```python
from build123d import *

# Parameters (mm, degrees)
BOSS_EXTRUDE1_DEPTH = 5
FILLET1_R           = 5
SKETCH2_R           = 1.3
CUT_EXTRUDE1_DEPTH  = 10
BOSS_EXTRUDE2_DEPTH = 45
BOSS_EXTRUDE3_DEPTH = 15
BOSS_EXTRUDE4_DEPTH = 6
BOSS_EXTRUDE5_START = -5.9
SKETCH6_R           = 4.9
SKETCH6_R_2         = 1.3
BOSS_EXTRUDE5_DEPTH = 5.9
BOSS_EXTRUDE6_DEPTH = 4
BOSS_EXTRUDE7_DEPTH = 5
BOSS_EXTRUDE8_DEPTH = 9
CHAMFER1_SIZE       = 5
FILLET2_R           = 6
SKETCH11_R          = 1.6
CUT_EXTRUDE2_DEPTH  = 10
FILLET3_R           = 10


# Some blends are built 0.0001 mm under size
with BuildPart() as part:
    # Sketch1 → Boss-Extrude1 (new body)
    with BuildSketch(Plane(origin=(0, 0, 0), x_dir=(1, 0, 0), z_dir=(0, 1, 0))):
        Polygon((4.09199016, 5.61187779), (0, 10), (0, 1.796035233), align=None)
        Polygon((0, 1.796035233), (0, 10), (-42.418514694, -29.555904884), (-38.326524534, -33.944027093), (-1.926011986, 0), align=None)
        Polygon((42, 10), (0, 10), (4.09199016, 5.61187779), (0, 1.796035233), (0, 0), (42, 0), align=None)
        Polygon((0, 0), (0, 1.796035233), (-1.926011986, 0), align=None)
    extrude(amount=BOSS_EXTRUDE1_DEPTH)

    # Fillet1
    fillet1_edges = [part.edges().sort_by_distance(p)[0] for p in [
        (42, 2.5, 0),
        (42, 2.5, -10),
    ]]
    fillet(fillet1_edges, radius=FILLET1_R - 0.0001)  # a hair under: the kernel refuses the full size

    # Sketch2 → Cut-Extrude1 (cut)
    with BuildSketch(Plane(origin=(0, 5, 0), x_dir=(1, 0, 0), z_dir=(0, 1, 0))):
        with Locations(Location((37, 5, 0), (0, 0, 270))):
            Circle(SKETCH2_R)
    extrude(amount=-CUT_EXTRUDE1_DEPTH, mode=Mode.SUBTRACT)

    # Sketch3 → Boss-Extrude2 (add)
    with BuildSketch(Plane(origin=(0, 5, 0), x_dir=(1, 0, 0), z_dir=(0, 1, 0))):
        Polygon((-42.418514694, -29.555904884), (-38.326524534, -33.944027093), (-20.12626826, -16.972013547), (-24.21825842, -12.583891337), align=None)
    extrude(amount=BOSS_EXTRUDE2_DEPTH)

    # Sketch4 → Boss-Extrude3 (add)
    with BuildSketch(Plane.XZ):
        Polygon((-42.418514694, 29.555904884), (-38.326524534, 33.944027093), (-20.12626826, 16.972013547), (-24.21825842, 12.583891337), align=None)
    extrude(amount=BOSS_EXTRUDE3_DEPTH)

    # Sketch5 → Boss-Extrude4 (add)
    with BuildSketch(Plane(origin=(-4.987820251, 0, -5.348782369), x_dir=(-0.7313537016191739, 0, 0.6819983600624947), z_dir=(-0.6819983600624948, 0, -0.731353701619174))):
        Polygon((26.294306197, -15), (26.294306197, 0), (13.888976828, 0), align=None)
        Polygon((13.888976828, 5), (26.294306197, 50), (26.294306197, 5), align=None)
    extrude(amount=-BOSS_EXTRUDE4_DEPTH)

    # Sketch6 → Boss-Extrude5 (add)
    with BuildSketch(Plane.XZ.offset(BOSS_EXTRUDE5_START)):
        with Locations(Location((37, -5, 0), (0, 0, 270))):
            Circle(SKETCH6_R)
        with Locations(Location((37, -5, 0), (0, 0, 90))):
            Circle(SKETCH6_R_2, mode=Mode.SUBTRACT)
    extrude(amount=BOSS_EXTRUDE5_DEPTH)

    # Sketch8 → Boss-Extrude6 (add)
    with BuildSketch(Plane.XZ):
        Polygon((0, -10), (-19.681916643, 8.353684194), (-15.589926483, 12.741806404), (8.797675114, -10), align=None)
    extrude(amount=BOSS_EXTRUDE6_DEPTH)

    # Sketch10 → Boss-Extrude7 (add)
    with BuildSketch(Plane(origin=(0, 5, 0), x_dir=(1, 0, 0), z_dir=(0, 1, 0))):
        Polygon((8.797675114, 10), (8.797675114, 0), (-1.926011986, 0), (-16.799617624, -13.869861642), (-20.891607784, -9.481739432), (0, 10), align=None)
    extrude(amount=BOSS_EXTRUDE7_DEPTH)

    # Sketch9 → Boss-Extrude8 (add)
    with BuildSketch(Plane(origin=(0, 5, 0), x_dir=(1, 0, 0), z_dir=(0, 1, 0))):
        Polygon((17.950520425, 10), (8.797675114, 10), (-1.926011986, 0), (8.797675114, 0), (17.950520425, 0), align=None)
    extrude(amount=-BOSS_EXTRUDE8_DEPTH)

    # Chamfer1
    # the kernel refuses this chamfer: 5 mm, written as the material it adds along each edge
    # the kernel refuses this chamfer: 5 mm, written as the material it takes off along each edge
    with BuildSketch(Plane(origin=(17.950520425, -4, 12.85841494), x_dir=(0.027495876610586317, 0.9996219169112968, 0), z_dir=(0, 0, -1))) as chamfer1_2_piece_1_section:
        Polygon((CHAMFER1_SIZE * 0.999621916911, -CHAMFER1_SIZE * 0.0274958766106), (-CHAMFER1_SIZE * 0.0274958766106, -CHAMFER1_SIZE * 0.999621916911), (0, 0), align=None)
    chamfer1_2_piece_1 = extrude(amount=35.71682988, mode=Mode.PRIVATE)
    chamfer1_2_piece_1 = split(chamfer1_2_piece_1, bisect_by=Plane(origin=(16.228298203, 0, -5), z_dir=(0, -1, 0)), keep=Keep.TOP, mode=Mode.PRIVATE)
    add(chamfer1_2_piece_1, mode=Mode.SUBTRACT)

    # Fillet2
    fillet2_edges = [part.edges().sort_by_distance(p)[0] for p in [
        (12.950520425, -4, -5),
        (16.950520425, 0, -5),
    ]]
    fillet(fillet2_edges, radius=FILLET2_R)

    # Sketch11 → Cut-Extrude2 (cut)
    with BuildSketch(Plane(origin=(0, 5, 0), x_dir=(1, 0, 0), z_dir=(0, 1, 0))):
        with Locations(Location((13.5, 5, 0), (0, 0, 270))):
            Circle(SKETCH11_R)
    extrude(amount=-CUT_EXTRUDE2_DEPTH, mode=Mode.SUBTRACT)

    # Fillet3
    fillet3_edges = [part.edges().sort_by_distance(p)[0] for p in [
        (-14.107655737, 10, 7.257584188),
        (-1.926011986, 3, 0),
        (0, 3, -10),
        (-15.518962067, -4, 8.573648632),
    ]]
    fillet(fillet3_edges, radius=FILLET3_R)


solid = part.part
```
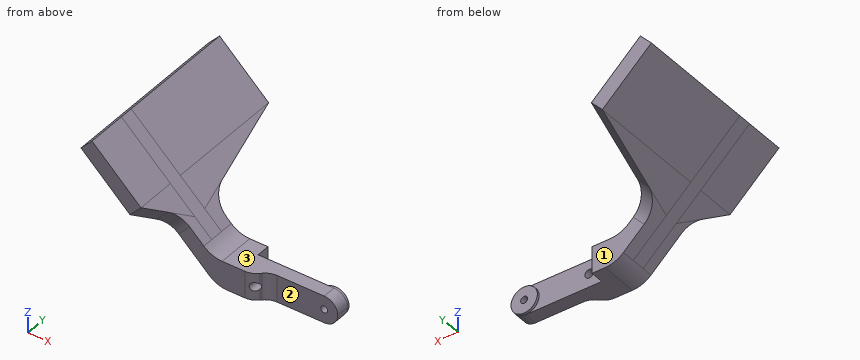
The model under review builds one solid part; all positions refer to its coordinate system, in mm. Face numbers are marked on the shaded views. A direction names the side the tool comes from. Give positions to 0.01 mm unless a question says otherwise; leave off trailing zeros. Loops run counter-clockwise (first coordinate to the right, second up) from the corner with the lowest first, then second, coordinate; pieces in that order, holes last. Notation, with made-up numbers: (36, 68) -> (40, 68) arc R21 ccw to (40, 101) -> close; hole circle Ø1 at (9, 14). An arc over 180 degrees is marked (long way). Use CSV: the item, a comma, the result in double quotes.
1. Consider section B-B, the plane z = 14.5. Write out the cut boundary in (x, y), then the cut area to 3 significant figures.
Result:
outline,"(-26.27, -15) -> (-22.43, -15) -> (-17.48, -10.62) -> (-17.48, 36.85) -> (-22.43, 50) -> (-26.27, 50) -> close"
area,"528 mm²"
2. Machinability: for the marked faces 1, 2 and 3, which of the approach directions +Z, -Z, +X, -X, +Y, -Y give a long, thin tool a straight path to every point of the face, cutting with its end or side? Answer none if there is none.
Result:
face 1,"-Z, +X, +Y"
face 2,"+Z, -Z, +X, -Y"
face 3,"+Z, +X, +Y, -Y"
3. Consider section A-A, the plane x = 13.5. Write out the cut boundary in (y, z), then the cut area to 3 significant figures.
Result:
outline,"(-3.18, -10) -> (5, -10) -> (5, -6.6) -> (-3.18, -6.6) -> close; (-3.18, -3.4) -> (5, -3.4) -> (5, 0) -> (-3.18, 0) -> close"
area,"55.6 mm²"
4. For P1, Ø9, axis at x = 1, z = -1.5, coming from the -Y side; P2, Ø3, axis at x = 30.5, z = -6, coming from the -Y side; P3, Ø2.5, axis at x = 37, z = -5, coming from the +Y side; P4, Ø8, axis at x = 23.5, z = -6, coming from the +Y side, all flat-tipped, find the tip position at first contact; note any pin that passes through.
Result:
P1,"stops at y = -4"
P2,"stops at y = 0"
P3,"passes through"
P4,"stops at y = 5"
5. Consider section C-C, the plane y = 15.5. Write out the cut boundary in (x, z), then the cut area to 3 significant figures.
Result:
outline,"(-42.42, 29.56) -> (-17.11, 5.96) -> (-13.02, 10.35) -> (-38.33, 33.94) -> close"
area,"208 mm²"
6. Consider section D-D, the plane x = 29. Write out the cut boundary in (y, z), then the cut area to 3 significant figures.
Result:
outline,"(0, -10) -> (5, -10) -> (5, 0) -> (0, 0) -> close"
area,"50.0 mm²"
7. To check wall thickness, follow probe 1 along Z at (x, y) = (37, 3.8); probe 2 along X at (y, z) = (3.2, -5); probe 3 along Z at (x, y) = (13.5, 0.5). State the ranges of each line that lie inside material, in increasing order. Write a range as from..to.
Result:
probe 1,"z = -10..-6.3, -3.7..0"
probe 2,"x = -5.36..11.9, 15.1..35.7, 38.3..42"
probe 3,"z = -10..-6.6, -3.4..0"
